The listing builds one solid part. Answer for the finished solid, in the listing's coordinates (mm). A direction names the side the tool comes from. Give positions to 0.01 mm unless a question says otherwise; leave off trailing zeros. Write each loop counter-clockwise with the first axis right and the second up, starting at its lowest first coordinate (ties: lowest second). Pieces come first, ordered by that corner, then holes. Notation, with made-up numbers: (-14.75, 15) -> (16.25, 15) arc R20 cw to (16.25, 53) -> close; hole circle Ø10 at (-21, 41). An arc over 180 degrees is marked (long way). Use CSV: the item, a comma, the result in double quotes. Start each with the question number.
from build123d import *

# Parameters (mm, degrees)
BOSS_EXTRUDE1_DEPTH = 5
CIRPATTERN1_COUNT   = 8
SKETCH2_R           = 2.443200814
BOSS_EXTRUDE2_DEPTH = 5


with BuildPart() as part:
    # Sketch1 → Boss-Extrude1 (new body)
    with BuildSketch(Plane.XY.offset(5)):
        with BuildLine():
            Line((0.41659025, 2.407422435), (0.640908077, 3.703726823))
            add(Edge.make_bspline(
                [(0.640908077, 3.703726823), (0.680350197, 4.297153912), (0.071093186, 4.99949455)],
                knots=[0.50407462, 0.50407462, 0.50407462, 1.738238777, 1.738238777, 1.738238777], degree=2, weights=[1, 0.815570405, 1]))
            ThreePointArc((0.071093186, 4.99949455), (0, 5), (-0.071093186, 4.99949455))
            add(Edge.make_bspline(
                [(-0.071093186, 4.99949455), (-0.684119659, 4.29533983), (-0.640908077, 3.703726823)],
                knots=[4.493136736, 4.493136736, 4.493136736, 5.781201385, 5.781201385, 5.781201385], degree=2, weights=[1, 0.799681158, 1]))
            Line((-0.640908077, 3.703726823), (-0.41659025, 2.407422435))
            Line((-0.41659025, 2.407422435), (0.41659025, 2.407422435))
        make_face()
    extrude(amount=-BOSS_EXTRUDE1_DEPTH)


with BuildPart() as cirpattern1_1:
    # CirPattern1: pattern copy
    add(part.part.rotate(Axis((0, 0, 0), (0, 0, 1)), 1 * 360 / CIRPATTERN1_COUNT))


with BuildPart() as cirpattern1_2:
    # CirPattern1: pattern copy
    add(part.part.rotate(Axis((0, 0, 0), (0, 0, 1)), 2 * 360 / CIRPATTERN1_COUNT))


with BuildPart() as cirpattern1_3:
    # CirPattern1: pattern copy
    add(part.part.rotate(Axis((0, 0, 0), (0, 0, 1)), 3 * 360 / CIRPATTERN1_COUNT))


with BuildPart() as cirpattern1_4:
    # CirPattern1: pattern copy
    add(part.part.rotate(Axis((0, 0, 0), (0, 0, 1)), 4 * 360 / CIRPATTERN1_COUNT))


with BuildPart() as cirpattern1_5:
    # CirPattern1: pattern copy
    add(part.part.rotate(Axis((0, 0, 0), (0, 0, 1)), 5 * 360 / CIRPATTERN1_COUNT))


with BuildPart() as cirpattern1_6:
    # CirPattern1: pattern copy
    add(part.part.rotate(Axis((0, 0, 0), (0, 0, 1)), 6 * 360 / CIRPATTERN1_COUNT))


with BuildPart() as cirpattern1_7:
    # CirPattern1: pattern copy
    add(part.part.rotate(Axis((0, 0, 0), (0, 0, 1)), 7 * 360 / CIRPATTERN1_COUNT))


with BuildPart() as part_1:
    add(part.part)

    add(cirpattern1_1.part)  # Boss-Extrude2 merges CirPattern1_1

    add(cirpattern1_2.part)  # Boss-Extrude2 merges CirPattern1_2

    add(cirpattern1_3.part)  # Boss-Extrude2 merges CirPattern1_3

    add(cirpattern1_4.part)  # Boss-Extrude2 merges CirPattern1_4

    add(cirpattern1_5.part)  # Boss-Extrude2 merges CirPattern1_5

    add(cirpattern1_6.part)  # Boss-Extrude2 merges CirPattern1_6

    add(cirpattern1_7.part)  # Boss-Extrude2 merges CirPattern1_7
    # Sketch2 → Boss-Extrude2 (add)
    with BuildSketch(Plane.XY.offset(5)):
        Circle(SKETCH2_R)
    extrude(amount=-BOSS_EXTRUDE2_DEPTH)


solid = part_1.part
Q1. For faces 4 (the face through (-1.781, 2.527, 2.535)), 5 (the face through (2.54, -1.79, 2.54)), 6 (the face through (1.781, -2.527, 2.535)), 7 (the face through (-2.54, 1.79, 2.54)), 8 (the face through (2.26, 0.93, 2.54)), determine the directions among +Z, -Z, +X, -X, +Y, -Y from which every point of the face is accessible in a straight line to the end or side of a thin tool.
Q2. Straight lines are drawn through the part: L1, parallel to Y at x = -2.25, z = 2.45; L2, parallel to X at y = -3, z = 0.65; L3, parallel to X at y = -2.5, z = 3.6. For each, find the intervals that lie inside material, in ascending order.
Q3. Flat-ended cylindrical pins translate along their axes: pin 1 Ø1.5 at (x, z) = (-2, 1) entering from -Y; pin 2 Ø6 at (x, y) = (-1.5, 1) entering from -Z. Find the tip coordinate at first contact, or state that the pin passes through.
Q4. Section B-B on y = -1 is taken. Give the vertices of the cut face in (x, z).
Q5. The mould has two halves that part along Y. Classify faces 1 (the face through (1.79, 2.54, 2.54)), 2 (the face through (-1.79, -2.54, 2.54)), 3 (the face through (-0.527, -3.047, 2.535)): +Y half, -Y half, draft (parallel to the pull), parting line (faces both ways), or undercut.
Q6. Section C-C on y = 1.25 is taken. Give the vertices of the cut face in (x, z), then the cut area to 3 significant figures.
Q7. Section A-A on y = 3.25 is taken. State how many separate pieces and enclosed holes the cut face has, then the cut area to 3 significant figures.
Output:
1,face 4,"+Z, -Z, +Y"
1,face 5,"+Z, -Z, +X"
1,face 6,"+Z, -Z, -Y"
1,face 7,"+Z, -Z, -X"
1,face 8,"+Z, -Z"
2,L1,"-3.16 to -1.59, -0.95 to 0.95, 1.59 to 3.16"
2,L2,"-3.51 to -2.11, -0.52 to 0.52, 2.11 to 3.51"
2,L3,"-3.32 to -1.76, -0.43 to 0.43, 1.76 to 3.32"
3,pin 1,"y = -3.43"
3,pin 2,"z = 0"
4,outline,"(-2.23, 0) -> (2.23, 0) -> (2.23, 5) -> (-2.23, 5) -> close"
5,face 1,"+Y half"
5,face 2,"-Y half"
5,face 3,"undercut"
6,outline,"(-2.1, 0) -> (2.1, 0) -> (2.1, 5) -> (-2.1, 5) -> close"
6,area,"21.0 mm²"
7,separate pieces,"3"
7,enclosed holes,"0"
7,area,"17.4 mm²"
